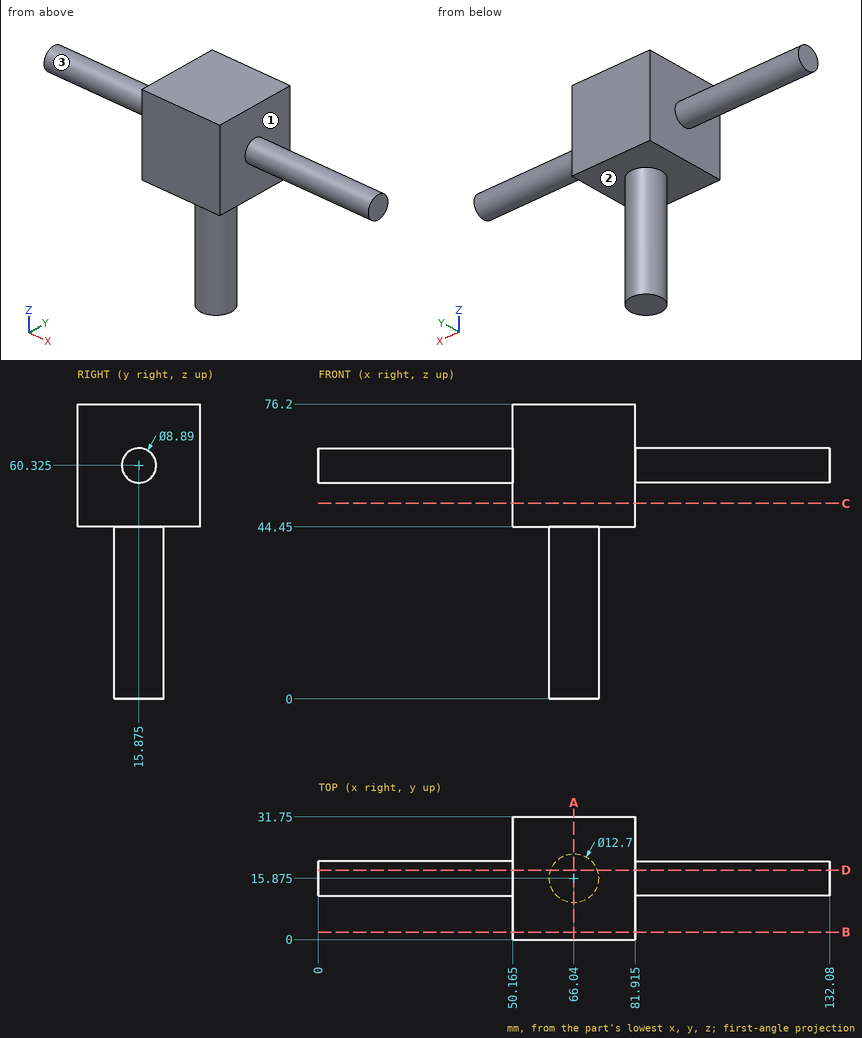
For this review, use the dimensioned drawing (mm, ordinates from the lowest corner) and the shaded views. A direction names the side the tool comes from. Coordinates: 2 decimals unless noted, no trailing zeros. Order: outer loops, then holes, each group sorted by start corner. A loop starts at its lowest first (then second) coordinate and runs counter-clockwise, first axis right, second up. Notation, with made-up numbers: (25, 29.5) -> (38, 29.5) arc R19 ccw to (38, 59.5) -> close; hole circle Ø6 at (54, -13.5). An arc over 180 degrees is marked (long way). One line per item, written item: value. Start each with the question number.
Q1. Insertion check: pin 1 Ø2 at (y, z) = (12.5, 8.5) entering from +X; pin 2 Ø4 at (y, z) = (10, 19.5) entering from +X; pin 3 Ø10 at (x, z) = (32, 57.5) entering from -Y; pin 4 Ø4 at (x, z) = (110, 68) entering from +Y. Each pin has a flat end and moves straight along its axis. Give the tip position at first contact, or say it passes through.
Q2. Take a section at B-B, the plane y = 2. State the section outline as (x, z) points (3 decimals), then the cut area to 3 significant figures.
Q3. Take a section at D-D, the plane y = 18. State the section outline as (x, z) points (3 decimals), then the cut area to 3 significant figures.
Q4. Take a section at C-C, the plane z = 50.5. State the section outline as (x, y) points (3 decimals), then the cut area to 3 significant figures.
Q5. For probe 1 along Z at (x, y) = (74.5, 16); probe 2 along X at (y, z) = (16, 34); probe 3 along X at (y, z) = (3, 67.5) (3 decimals), list the stretches that pass through material, from the lowest coordinate up.
Q6. Take a section at A-A, the plane x = 66.04. State the section outline as (y, z) points (3 decimals), then the cut area to 3 significant figures.
Q7. Tool access review of the marked faces 1, 2 and 3: name each direction out of +Z, -Z, +X, -X, +Y, -Y from which nothing blocks a thin tool from reaching the whole face with its end or side.
Values follow:
1. pin 1: stops at x = 71.93
1. pin 2: stops at x = 71.07
1. pin 3: stops at y = 11.43
1. pin 4: passes through
2. outline: (50.165, 44.45) -> (81.915, 44.45) -> (81.915, 76.2) -> (50.165, 76.2) -> close
2. area: 1,010 mm2
3. outline: (0, 56.421) -> (50.165, 56.421) -> (50.165, 44.45) -> (60.056, 44.45) -> (60.056, 0) -> (72.024, 0) -> (72.024, 44.45) -> (81.915, 44.45) -> (81.915, 56.421) -> (132.08, 56.421) -> (132.08, 64.229) -> (81.915, 64.229) -> (81.915, 76.2) -> (50.165, 76.2) -> (50.165, 64.229) -> (0, 64.229) -> close
3. area: 2,320 mm2
4. outline: (50.165, 0) -> (81.915, 0) -> (81.915, 31.75) -> (50.165, 31.75) -> close
4. area: 1,010 mm2
5. probe 1: z = 44.45 to 76.2
5. probe 2: x = 59.69 to 72.39
5. probe 3: x = 50.165 to 81.915
6. outline: (0, 44.45) -> (9.525, 44.45) -> (9.525, 0) -> (22.225, 0) -> (22.225, 44.45) -> (31.75, 44.45) -> (31.75, 76.2) -> (0, 76.2) -> close
6. area: 1,570 mm2
7. face 1: +X
7. face 2: -Z
7. face 3: -X
